Design review of the part built by this model. Coordinates are the model's own, in mm. A direction names the side the tool comes from. Coordinates: 2 decimals unless noted, no trailing zeros. Order: outer loops, then holes, each group sorted by start corner. A loop starts at its lowest first (then second) coordinate and runs counter-clockwise, first axis right, second up. Notation, with made-up numbers: (76.5, 5) -> (87.5, 5) arc R16 cw to (87.5, 21) -> close; hole circle Ø9 at (78, 29.25). An arc over 180 degrees is marked (long way). Use a Markdown table: item, result. Add a question column.
Q1. Add section C-C (z = -30). State the section outline as (x, y) points, then the cut area to 3 significant figures.
Q2. The part is to be moulded in two halves that separate along Z. For faces 6 (the face through (3, 14, -51.562)), 7 (the face through (34, 1, 8.89)), 8 (the face through (36.322, 14, -36)), 9 (the face through (38.1, 15, -31)), say which applies: pulls with the +Z half, pulls with the -Z half, needs draft (parallel to the pull), parting line crosses it, or undercut.
Q3. Wall thickness on probe 1 along Z at (x, y) = (17, 25); probe 2 along X at (y, z) = (15.5, -3.5); probe 3 along Z at (x, y) = (19.5, 1): over which ranges is each line inside the solid? List them lowest first.
Q4. Add section A-A (y = 5). State the section outline as (x, z) points, then the cut area to 3 significant figures.
Q5. Add section D-D (y = 17.5). State the section outline as (x, z) points.
Q6. Machinability: for faces 1 (the face through (1, 11, -5.08)), 2 (the face through (25.908, 1, 4)), 3 (the face through (17.018, 2, 1)), 4 (the face through (2.54, 15, -63)), 5 (the face through (21, 14, -70.612)), which of the approach directions +Z, -Z, +X, -X, +Y, -Y give a long, thin tool a straight path to every point of the face, cutting with its end or side? Answer none if there is none.
Q7. Insertion check: pin 1 (0.5 mm diameter, centred on x = 0.5, y = 12, fed in from -Z); pin 2 (1.3 mm diameter, centred on y = 1.5, z = 4, fed in from -X); pin 3 (2.5 mm diameter, centred on x = 35, z = 2.5, fed in from +Y). Each pin has a flat end and moves straight along its axis. Give the tip position at first contact, or say it passes through.
Q8. Add section B-B (x = 31). State the section outline as (y, z) points, then the cut area to 3 significant figures.
from build123d import *

# Parameters (mm, degrees)
BOSS_EXTRUDE1_DEPTH = 30.48
SHELL1_T            = -1.778
CUT_EXTRUDE3_REACH  = 89.298
SKETCH7_W           = 15.24
SKETCH7_H           = 10.16
SKETCH2_W           = 8.89
SKETCH2_H           = 2.54
BOSS_EXTRUDE2_DEPTH = 8.89
SKETCH3_R           = 1.55
CUT_EXTRUDE1_DEPTH  = 87.444003262
SKETCH4_R           = 1.55
CUT_EXTRUDE2_DEPTH  = 87.444003262
SKETCH8_W           = 43.18
SKETCH8_H           = 22.86
CUT_EXTRUDE4_DEPTH  = 11.684


with BuildPart() as part:
    # Sketch1 → Boss-Extrude1 (new body)
    with BuildSketch(Plane(origin=(0, 0, 0), x_dir=(1, 0, 0), z_dir=(0, 1, 0))):
        Polygon((0, 0), (38.1, 0), (38.1, 53.34), (38.1, 72.39), (2.54, 72.39), (2.54, 53.34), (0, 53.34), align=None)
    extrude(amount=BOSS_EXTRUDE1_DEPTH)

    # Shell1
    shell1_openings = [part.faces().sort_by_distance(p)[0] for p in [
        (19.3675, 0, -35.71875),
    ]]
    offset(amount=SHELL1_T, openings=shell1_openings, kind=Kind.INTERSECTION)

    # Sketch7 → Cut-Extrude3 (cut, up to next)
    with BuildSketch(Plane.XY, mode=Mode.PRIVATE) as cut_extrude3_sk1:
        with Locations((9.398, 5.08)):
            Rectangle(SKETCH7_W, SKETCH7_H)
    cut_extrude3_tool1 = extrude(cut_extrude3_sk1.sketch, amount=-CUT_EXTRUDE3_REACH, mode=Mode.PRIVATE) & part.part
    add(cut_extrude3_tool1.solids().sort_by_distance((9.398, 5.08, 0))[0], mode=Mode.SUBTRACT)

    # Sketch2 → Boss-Extrude2 (add)
    with BuildSketch(Plane.XY):
        with Locations((21.463, 1.27)):
            Rectangle(SKETCH2_W, SKETCH2_H)
        with Locations((33.655, 1.27)):
            Rectangle(SKETCH2_W, SKETCH2_H)
    extrude(amount=BOSS_EXTRUDE2_DEPTH)

    # Sketch3 → Cut-Extrude1 (cut, through all)
    with BuildSketch(Plane(origin=(0, 2.54, 0), x_dir=(1, 0, 0), z_dir=(0, 1, 0))):
        with Locations(Location((21.463, -4.445, 0), (0, 0, 270))):
            Circle(SKETCH3_R)
    extrude(amount=-CUT_EXTRUDE1_DEPTH, mode=Mode.SUBTRACT)

    # Sketch4 → Cut-Extrude2 (cut, through all)
    with BuildSketch(Plane(origin=(0, 2.54, 0), x_dir=(1, 0, 0), z_dir=(0, 1, 0))):
        with Locations(Location((33.655, -4.445, 0), (0, 0, 180))):
            Circle(SKETCH4_R)
    extrude(amount=-CUT_EXTRUDE2_DEPTH, mode=Mode.SUBTRACT)

    # Sketch8 → Cut-Extrude4 (cut)
    with BuildSketch(Plane.ZY):
        with Locations((-26.67, 11.43)):
            Rectangle(SKETCH8_W, SKETCH8_H)
    extrude(amount=-CUT_EXTRUDE4_DEPTH, mode=Mode.SUBTRACT)


solid = part.part
Established:
| question | item | result |
|---|---|---|
| 1 | outline | (0, 22.86) -> (1.78, 22.86) -> (1.78, 28.7) -> (36.32, 28.7) -> (36.32, 0) -> (38.1, 0) -> (38.1, 30.48) -> (0, 30.48) -> close |
| 1 | area | 129 mm^2 |
| 2 | face 6 | undercut |
| 2 | face 7 | pulls with the +Z half |
| 2 | face 8 | undercut |
| 2 | face 9 | needs draft |
| 3 | probe 1 | -72.39 to -70.61, -1.78 to 0 |
| 3 | probe 2 | 0 to 1.78, 36.32 to 38.1 |
| 3 | probe 3 | -72.39 to -70.61, -1.78 to 8.89 |
| 4 | outline | (0, -53.34) -> (2.54, -53.34) -> (2.54, -72.39) -> (38.1, -72.39) -> (38.1, 0) -> (17.02, 0) -> (17.02, -1.78) -> (36.32, -1.78) -> (36.32, -70.61) -> (4.32, -70.61) -> (4.32, -51.56) -> (1.78, -51.56) -> (1.78, -48.26) -> (0, -48.26) -> close; (0, -5.08) -> (1.78, -5.08) -> (1.78, 0) -> (0, 0) -> close |
| 4 | area | 276 mm^2 |
| 5 | outline | (0, -53.34) -> (2.54, -53.34) -> (2.54, -72.39) -> (38.1, -72.39) -> (38.1, 0) -> (0, 0) -> (0, -5.08) -> (1.78, -5.08) -> (1.78, -1.78) -> (36.32, -1.78) -> (36.32, -70.61) -> (4.32, -70.61) -> (4.32, -51.56) -> (1.78, -51.56) -> (1.78, -48.26) -> (0, -48.26) -> close |
| 6 | face 1 | -X, -Y |
| 6 | face 2 | +Z, +Y, -Y |
| 6 | face 3 | +Z, -Y |
| 6 | face 4 | -Z, -X, +Y, -Y |
| 6 | face 5 | -Y |
| 7 | pin 1 | z = -53.34 |
| 7 | pin 2 | x = 17.02 |
| 7 | pin 3 | y = 2.54 |
| 8 | outline | (0, -72.39) -> (30.48, -72.39) -> (30.48, 0) -> (2.54, 0) -> (2.54, 8.89) -> (0, 8.89) -> (0, -1.78) -> (28.7, -1.78) -> (28.7, -70.61) -> (0, -70.61) -> close |
| 8 | area | 253 mm^2 |
